Can you work these out from the model? Positions are in its coordinate system, mm. A direction names the side the tool comes from. Give positions to 0.01 mm unless a question says otherwise; leave off trailing zeros. Order: outer loops, then holes, each group sorted by start corner. A loop starts at its lowest first (then second) coordinate and runs counter-clockwise, first axis right, second up. Notation, with made-up numbers: (64, 69) - (108, 69) arc R19 ccw to (108, 73) - close; hole circle Ø9 at (75, 48.5). An arc over 180 degrees is marked (long way). Return JSON: item names as keys, results as strings.
```python
from build123d import *

# Parameters (mm, degrees)
F0_W     = 50
F0_H     = 35
F0_R     = 11.05
F1_DEPTH = 36
F2_D     = 3.2
F2_DEPTH = 12
F2_TIP   = 0.9613769904
F3_SIZE  = 1
F5_D     = 4.2
F5_DEPTH = 12
F5_TIP   = 1.2618073


with BuildPart() as f1:
    # F0 (on Front) → F1 (new body)
    with BuildSketch(Plane.XZ):
        with Locations((0, -0.2)):
            Rectangle(F0_W, F0_H)
        Circle(F0_R, mode=Mode.SUBTRACT)
    extrude(amount=F1_DEPTH)

    # F2
    with Locations(Plane(origin=(0, 0, 0), x_dir=(1, 0, 0), z_dir=(0, 1, 0))):
        with Locations((-12.3743686708, -12.3743686708), (-17.5, 0), (-12.3743686708, 12.3743686708), (12.3743686708, 12.3743686708), (17.5, 0), (12.3743686708, -12.3743686708)):
            Hole(F2_D / 2, depth=F2_DEPTH)
            with Locations((0, 0, -(F2_DEPTH + F2_TIP / 2))):  # 118° drill point
                Cone(0, F2_D / 2, F2_TIP, mode=Mode.SUBTRACT)

    # F3
    f3_edges = [f1.edges().sort_by_distance(p)[0] for p in [
        (25, -18, 17.3),
        (0, 0, 17.3),
        (-25, -18, 17.3),
        (0, -36, 17.3),
    ]]
    chamfer(f3_edges, length=F3_SIZE)

    # F5
    with Locations(Plane(origin=(0, 0, -17.7), x_dir=(1, 0, 0), z_dir=(0, 0, -1))):
        with Locations((17.5, 6), (17.5, 30), (-17.5, 30), (-17.5, 6)):
            Hole(F5_D / 2, depth=F5_DEPTH)
            with Locations((0, 0, -(F5_DEPTH + F5_TIP / 2))):  # 118° drill point
                Cone(0, F5_D / 2, F5_TIP, mode=Mode.SUBTRACT)


solid = f1.part
```
1. Suppose I cut it at C-C (y = -14). List the corners of the cut face in (x, z) for me, plus the area to 3 significant figures.
Checks:
{"outline": "(-25, -17.7) - (25, -17.7) - (25, 16.3) - (24, 17.3) - (-24, 17.3) - (-25, 16.3) - close; hole circle Ø22.1 at (0, 0)", "area": "1,370 mm^2"}
2. Suppose I cut it at D-D (x = 8.5). List the corners of the cut face in (y, z) for me, plus the area to 3 significant figures.
Checks:
{"outline": "(-36, -17.7) - (0, -17.7) - (0, -7.06) - (-36, -7.06) - close; (-36, 7.06) - (0, 7.06) - (0, 16.3) - (-1, 17.3) - (-35, 17.3) - (-36, 16.3) - close", "area": "751 mm^2"}
3. Suppose I cut it at A-A (x = 0). List the corners of the cut face in (y, z) for me, plus the area to 3 significant figures.
Checks:
{"outline": "(-36, -17.7) - (0, -17.7) - (0, -11.05) - (-36, -11.05) - close; (-36, 11.05) - (0, 11.05) - (0, 16.3) - (-1, 17.3) - (-35, 17.3) - (-36, 16.3) - close", "area": "463 mm^2"}
4. If I drill on L1, parallel to Y at x = 17.5, z = -11.25; L2, parallel to Z at x = -6, y = -23; L3, parallel to Z at x = 2.5, y = -33, over which ranges is the centre line in solid material (lowest first)? Write a range as [from, to].
Checks:
{"L1": "[-36, -32.1], [-27.9, -8.1], [-3.9, 0]", "L2": "[-17.7, -9.28], [9.28, 17.3]", "L3": "[-17.7, -10.76], [10.76, 17.3]"}
5. For pin 1 Ø1.9 at (x, z) = (12.37, 12.37) entering from +Y; pin 2 Ø2.5 at (x, z) = (-12.37, -12.37) entering from +Y; pin 3 Ø4 at (x, y) = (-17.5, -6) entering from -Z; pin 4 Ø10 at (x, z) = (0.5, 2) entering from -Y, each with a flat end and sliding along its axis, tell me the tip position at first contact or that it passes through.
Checks:
{"pin 1": "y = -12.39", "pin 2": "y = -12.21", "pin 3": "z = -5.64", "pin 4": "through"}
6. Suppose I cut it at B-B (z = -8). List the corners of the cut face in (x, y) for me, plus the area to 3 significant figures.
Checks:
{"outline": "(-25, -36) - (-7.62, -36) - (-7.62, 0) - (-25, 0) - close; (7.62, -36) - (25, -36) - (25, 0) - (7.62, 0) - close; hole circle Ø4.2 at (-17.5, -30); hole circle Ø4.2 at (-17.5, -6); hole circle Ø4.2 at (17.5, -30); hole circle Ø4.2 at (17.5, -6)", "area": "1,200 mm^2"}
7. On a 3-axis mill with a long thin cutter (end or side, diameter ignored), from which of +Z, -Z, +X, -X, +Y, -Y can I reach the whole of each face in a straight line? I mean faces 4 (the face through (-13.85, -6.08, -11.76)), 5 (the face through (25, -18, -1)), 6 (the face through (-18.469, -28.137, -11.616)). Say none if no direction works.
Checks:
{"face 4": "+Y", "face 5": "+Z, -Z, +X, +Y, -Y", "face 6": "-Z"}
8. Thinking about a two-plate mould opening in Z: for faces 1 (the face through (-12.435, -12.794, -12.103)), 2 (the face through (16.531, -28.137, -11.616)), 3 (the face through (17.136, -6.016, -4.657)), which applies, +Z half, -Z half, draft (parallel to the pull), parting line (faces both ways), or undercut?
Checks:
{"face 1": "undercut", "face 2": "draft", "face 3": "-Z half"}
